```python
from build123d import *

# Parameters (mm, degrees)
F0_W      = 35
F0_H      = 35
F1_DEPTH  = 1.5
F2_SIZE   = 6.1
F3_W      = 35
F3_H      = 35
F4_DEPTH  = 8
F5_SIZE   = 2.6
F7_DEPTH  = 9
F8_R      = 11
F9_DEPTH  = 2
F10_R     = 2.5
F11_DEPTH = 18
F12_R     = 1.5
F13_DEPTH = 6
F14_SIZE  = 0.5
F16_D     = 1
F16_DEPTH = 3
F16_TIP   = 0.3004303095


with BuildPart() as f1:
    # F0 (on Top) → F1 (new body, symmetric)
    with BuildSketch(Plane.XY):
        Rectangle(F0_W, F0_H)
    extrude(amount=F1_DEPTH, both=True)

    # F2
    f2_edges = [f1.edges().sort_by_distance(p)[0] for p in [
        (-17.5, -17.5, 0),
        (17.5, -17.5, 0),
        (17.5, 17.5, 0),
        (-17.5, 17.5, 0),
    ]]
    chamfer(f2_edges, length=F2_SIZE)

    # F3 (on face) → F4 (join)
    with BuildSketch(Plane.XY.offset(1.5)):
        Rectangle(F3_W, F3_H)
    extrude(amount=F4_DEPTH)

    # F5
    f5_edges = [f1.edges().sort_by_distance(p)[0] for p in [
        (-17.5, -17.5, 5.5),
        (17.5, -17.5, 5.5),
        (17.5, 17.5, 5.5),
        (-17.5, 17.5, 5.5),
    ]]
    chamfer(f5_edges, length=F5_SIZE)

    # F6 (on face) → F7 (join)
    with BuildSketch(Plane(origin=(0, 0, -1.5), x_dir=(1, 0, 0), z_dir=(0, 0, -1))):
        Polygon((-14.9, -17.5), (14.9, -17.5), (17.5, -14.9), (17.5, 14.9), (14.9, 17.5), (-14.9, 17.5), (-17.5, 14.9), (-17.5, -14.9), align=None)
    extrude(amount=F7_DEPTH)

    # F8 (on face) → F9 (join)
    with BuildSketch(Plane.XY.offset(9.5)):
        Circle(F8_R)
    extrude(amount=F9_DEPTH)

    # F10 (on face) → F11 (join)
    with BuildSketch(Plane.XY.offset(11.5)):
        Circle(F10_R)
    extrude(amount=F11_DEPTH)

    # F12 (on face) → F13 (cut)
    with BuildSketch(Plane.XY.offset(9.5)):
        with Locations((-13, 13)):
            Circle(F12_R)
        with Locations((13, 13)):
            Circle(F12_R)
        with Locations((-13, -13)):
            Circle(F12_R)
        with Locations((13, -13)):
            Circle(F12_R)
    extrude(amount=-F13_DEPTH, mode=Mode.SUBTRACT)

    # F14
    f14_edges = [f1.edges().sort_by_distance(p)[0] for p in [
        (-2.5, 0, 29.5),
    ]]
    chamfer(f14_edges, length=F14_SIZE)

    # F16
    with Locations(Plane.XY.offset(29.5)):
        with Locations((0, 0)):
            Hole(F16_D / 2, depth=F16_DEPTH)
            with Locations((0, 0, -(F16_DEPTH + F16_TIP / 2))):  # 118° drill point
                Cone(0, F16_D / 2, F16_TIP, mode=Mode.SUBTRACT)


solid = f1.part
```
The listing builds one solid part. Answer for the finished solid, in the listing's coordinates (mm). A direction names the side the tool comes from. Coordinates: 2 decimals unless noted, no trailing zeros. Loops run counter-clockwise (first coordinate to the right, second up) from the corner with the lowest first, then second, coordinate; pieces in that order, holes last. Notation, with made-up numbers: M 49,87 L 77,87 A30 cw 77,121 Z; hole C -2.75,22 d10. An arc over 180 degrees is marked long. Answer as a JSON object with one key per item and string values. Group by question number.
Item 1: Section A-A (y = 15.5) is taken. Write down the section's boundary in (x, z), and give its area (3 significant figures).
Item 2: Section B-B (x = -13) is taken. Write down the section's boundary in (y, z), and give its area (3 significant figures).
Item 3: Each of these flat-tipped pins is pushed along its axis until it touches: P1, Ø3, axis at y = 1.5, z = 17.5, coming from the +X side; P2, Ø1.8, axis at x = 14, y = -16, coming from the +Z side; P3, Ø0.9, axis at x = 13.5, y = 13, coming from the +Z side. Where does it stop, or does it pass through?
Item 4: Consider L1, parallel to Y at x = 13, z = 7.1; L2, parallel to Z at x = 2, y = -15; L3, parallel to Y at x = 1.5, z = 19. Determine where each line is inside the solid, lowest interval first.
Item 5: Which of the six approach directions +Z, -Z, +X, -X, +Y, -Y give full straight-line access (tool end or side, diameter ignored) to faces 1 (the face through (-14.5, 13.07, 6.54)), 2 (the face through (15, 15, -1.5)), 3 (the face through (15, -15, -1.5))?
Item 6: Determine the mould class of faces 4 (the face through (0, 0, -10.5)), 5 (the face through (-15, 15, -1.5)), 6 (the face through (-0.5, 0.5, 29.5)), 7 (the face through (-2.38, -10.74, 10.49)) for opening direction Z: +Z half, -Z half, draft (parallel to the pull), parting line (faces both ways), or undercut.
Item 7: Section D-D (x = 5) is taken. Write down the section's boundary in (y, z).
Solved:
{
 "1": {"outline": "M -16.9,-10.5 L 16.9,-10.5 L 16.9,-1.5 L 13.4,-1.5 L 13.4,1.5 L 16.9,1.5 L 16.9,9.5 L -16.9,9.5 L -16.9,1.5 L -13.4,1.5 L -13.4,-1.5 L -16.9,-1.5 Z", "area": "655 mm2"},
 "2": {"outline": "M -17.5,-10.5 L 17.5,-10.5 L 17.5,-1.5 L 15.9,-1.5 L 15.9,1.5 L 17.5,1.5 L 17.5,9.5 L 14.5,9.5 L 14.5,3.5 L 11.5,3.5 L 11.5,9.5 L -11.5,9.5 L -11.5,3.5 L -14.5,3.5 L -14.5,9.5 L -17.5,9.5 L -17.5,1.5 L -15.9,1.5 L -15.9,-1.5 L -17.5,-1.5 Z", "area": "654 mm2"},
 "3": {"P1": "stops at x = 2.5", "P2": "stops at z = 9.5", "P3": "stops at z = 3.5"},
 "4": {"L1": "y = -17.5 to -14.5, -11.5 to 11.5, 14.5 to 17.5", "L2": "z = -10.5 to 9.5", "L3": "y = -2 to 2"},
 "5": {"face 1": "+Z", "face 2": "+X, +Y", "face 3": "+X, -Y"},
 "6": {"face 4": "-Z half", "face 5": "undercut", "face 6": "+Z half", "face 7": "draft"},
 "7": {"outline": "M -17.5,-10.5 L 17.5,-10.5 L 17.5,9.5 L 9.8,9.5 L 9.8,11.5 L -9.8,11.5 L -9.8,9.5 L -17.5,9.5 Z"}
}
